```python
from build123d import *

# Parameters (mm, degrees)
ESTRUSIONE_ESTRUSIONE8_DEPTH = 2
SCHIZZO8_R                   = 4
TAGLIO_ESTRUSIONE6_DEPTH     = 2
SCHIZZO15_R                  = 4
TAGLIO_ESTRUSIONE7_DEPTH     = 2
SCHIZZO16_R                  = 4
TAGLIO_ESTRUSIONE9_DEPTH     = 2


with BuildPart() as part:
    # Schizzo2 → Estrusione-Estrusione8 (new body)
    with BuildSketch(Plane(origin=(0, 0, 0), x_dir=(1, 0, 0), z_dir=(0, 1, 0))):
        with BuildLine():
            Line((-6.935, -4.36), (-6.935, 0.81))
            ThreePointArc((-6.935, 0.81), (-6.495660172, 1.870660172), (-5.435, 2.31))
            Line((-5.435, 2.31), (5.435, 2.31))
            ThreePointArc((5.435, 2.31), (6.495660172, 1.870660172), (6.935, 0.81))
            Line((6.935, 0.81), (6.935, -4.36))
            Line((6.935, -4.36), (11.035, -4.36))
            Line((11.035, -4.36), (11.035, 4.36))
            Line((11.035, 4.36), (15.01, 11.03))
            Line((15.01, 11.03), (15.01, 15.13))
            Line((15.01, 15.13), (16.868239421, 16.905343982))
            Line((16.868239421, 16.905343982), (16.868239421, 17.200505886))
            ThreePointArc((16.868239421, 17.200505886), (16.721792811, 17.554059277), (16.368239421, 17.700505886))
            Line((16.368239421, 17.700505886), (-14.992624707, 17.700505886))
            Line((-14.992624707, 17.700505886), (-16.351038686, 17.700505886))
            ThreePointArc((-16.351038686, 17.700505886), (-16.704592076, 17.554059277), (-16.851038686, 17.200505886))
            Line((-16.851038686, 17.200505886), (-16.851038686, 16.905667142))
            Line((-16.851038686, 16.905667142), (-14.992624707, 15.130505886))
            Line((-14.992624707, 15.130505886), (-14.992624707, 11.030505886))
            Line((-14.992624707, 11.030505886), (-11.035, 4.36))
            Line((-11.035, 4.36), (-11.035, -4.36))
            Line((-11.035, -4.36), (-6.935, -4.36))
        make_face()
    extrude(amount=ESTRUSIONE_ESTRUSIONE8_DEPTH)

    # Schizzo8 → Taglio-Estrusione6 (cut)
    with BuildSketch(Plane(origin=(0, 0, 0), x_dir=(1, 0, 0), z_dir=(0, 1, 0))):
        with Locations((8.985, 13.08010159)):
            Circle(SCHIZZO8_R)
    extrude(amount=TAGLIO_ESTRUSIONE6_DEPTH, mode=Mode.SUBTRACT)

    # Schizzo15 → Taglio-Estrusione7 (cut)
    with BuildSketch(Plane(origin=(0, 0, 0), x_dir=(1, 0, 0), z_dir=(0, 1, 0))):
        with Locations((0.00688301, 13.08)):
            Circle(SCHIZZO15_R)
    extrude(amount=TAGLIO_ESTRUSIONE7_DEPTH, mode=Mode.SUBTRACT)

    # Schizzo16 → Taglio-Estrusione9 (cut)
    with BuildSketch(Plane(origin=(0, 0, 0), x_dir=(1, 0, 0), z_dir=(0, 1, 0))):
        with Locations((-8.985, 13.080505886)):
            Circle(SCHIZZO16_R)
    extrude(amount=TAGLIO_ESTRUSIONE9_DEPTH, mode=Mode.SUBTRACT)


solid = part.part
```
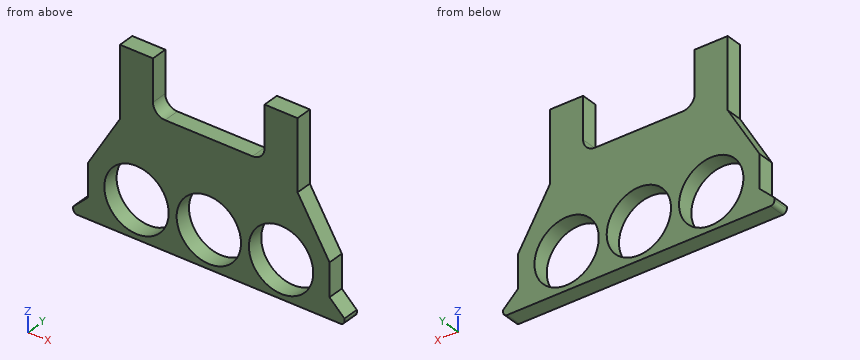
Geometry check sheet. Reference: the model listing, model coordinates, mm. Coordinates: 2 decimals unless noted, no trailing zeros. Write each loop counter-clockwise with the first axis right and the second up, starting at its lowest first coordinate (ties: lowest second). Pieces come first, ordered by that corner, then holes. Notation, with made-up numbers: (72.5, 17) -> (106.5, 17) arc R19 cw to (106.5, 50) -> close; hole circle Ø2 at (67.5, 70.25). An arc over 180 degrees is marked (long way). Use CSV: the item, a comma, the result in double quotes. Start each with the question number.
Item 1: Depth check by flat-ended pin: pin 1 Ø0.6 at (y, z) = (1.5, -13.5) entering from -X; pin 2 Ø1 at (y, z) = (1, 0) entering from -X (3 decimals). Enter the tip coordinate at first touch or a pass-through.
Item 2: Cross-section at A-A, the plane z = -10.25. Record the cut outline in (x, y), plus the area to 3 significant figures.
Item 3: Cross-section at B-B, the plane x = 1. Record the cut outline in (y, z).
Item 4: Cross-section at D-D, the plane x = -8.5. Record the cut outline in (y, z), plus the area to 3 significant figures.
Item 5: Thickness scan on line 1 (X direction, y = 1.3, z = -13.08) (3 decimals); line 2 (X direction, y = 0.65, z = -15.75); line 3 (X direction, y = 0.75, z = 2.5) (3 decimals). Record the ranges inside material, lowest first.
Item 6: Cross-section at C-C, the plane y = 1.15. State how many separate pieces and enclosed holes the cut face has, plus the area to 3 significant figures.
Answers:
1,pin 1,"x = -14.99"
1,pin 2,"x = -11.035"
2,outline,"(-14.53, 0) -> (-11.81, 0) -> (-11.81, 2) -> (-14.53, 2) -> close; (-6.16, 0) -> (-2.82, 0) -> (-2.82, 2) -> (-6.16, 2) -> close; (2.83, 0) -> (6.16, 0) -> (6.16, 2) -> (2.83, 2) -> close; (11.81, 0) -> (14.55, 0) -> (14.55, 2) -> (11.81, 2) -> close"
2,area,"24.2 mm^2"
3,outline,"(0, -17.7) -> (2, -17.7) -> (2, -16.95) -> (0, -16.95) -> close; (0, -9.21) -> (2, -9.21) -> (2, -2.31) -> (0, -2.31) -> close"
4,outline,"(0, -17.7) -> (2, -17.7) -> (2, -17.05) -> (0, -17.05) -> close; (0, -9.11) -> (2, -9.11) -> (2, 4.36) -> (0, 4.36) -> close"
4,area,"28.2 mm^2"
5,line 1,"-14.993 to -12.985, -4.985 to -3.993, 4.007 to 4.985, 12.985 to 15.01"
5,line 2,"-15.64 to -11.96, -6.01 to -2.97, 2.99 to 6.01, 11.96 to 15.66"
5,line 3,"-11.035 to -6.935, 6.935 to 11.035"
6,separate pieces,"1"
6,enclosed holes,"3"
6,area,"330 mm^2"
